The model under review builds one solid part; all positions refer to its coordinate system, in mm. Face numbers are marked on the shaded views. A direction names the side the tool comes from. Give positions to 0.01 mm unless a question says otherwise; leave off trailing zeros. Loops run counter-clockwise (first coordinate to the right, second up) from the corner with the lowest first, then second, coordinate; pieces in that order, holes last. Notation, with made-up numbers: (-3.75, -25) - (35.25, -25) arc R18 ccw to (35.25, 3) - close; hole circle Ø9 at (62.25, 27). An arc over 180 degrees is marked (long way). Answer as a JSON object with one key per item and string values.
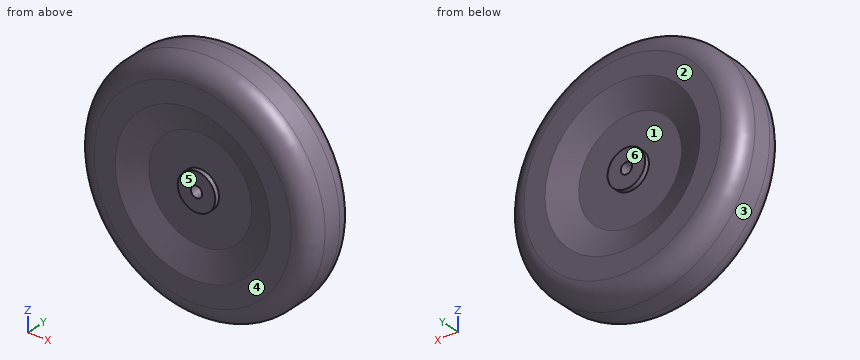
from build123d import *

# Parameters (mm, degrees)
F2_R = 20


with BuildPart() as f1:
    # F0 (on Right) → F1 (revolve)
    with BuildSketch(Plane.YZ):
        Polygon((-30, 82.617566), (-20, 54.791786), (-20, 20), (-25, 20), (-25, 6), (0, 6), (20, 6), (25, 6), (25, 20), (20, 20), (20, 54.791786), (30, 82.617566), (30, 125), (0, 125), (-30, 125), align=None)
    revolve(axis=Axis((0, 0.420819, 0), (0, 1, 0)))

    # F2
    f2_edges = [f1.edges().sort_by_distance(p)[0] for p in [
        (0, -30, -125),
        (0, 30, -125),
    ]]
    fillet(f2_edges, radius=F2_R)


solid = f1.part
Q1. The part is to be moulded in two halves that separate along X. For the marked faces 1, 2 and 3, say which applies: +X half, -X half, draft (parallel to the pull), parting line (faces both ways), or undercut.
Results:
{"face 1": "undercut", "face 2": "draft", "face 3": "parting line"}
Q2. Consider section A-A, the plane x = 0. State the section outline as (y, z) points, plus the area to 3 significant figures.
Results:
{"outline": "(-30, -105) arc R20 ccw to (-10, -125) - (10, -125) arc R20 ccw to (30, -105) - (30, -82.62) - (20, -54.79) - (20, -20) - (25, -20) - (25, -6) - (-25, -6) - (-25, -20) - (-20, -20) - (-20, -54.79) - (-30, -82.62) - close; (-30, 82.62) - (-20, 54.79) - (-20, 20) - (-25, 20) - (-25, 6) - (25, 6) - (25, 20) - (20, 20) - (20, 54.79) - (30, 82.62) - (30, 105) arc R20 ccw to (10, 125) - (-10, 125) arc R20 ccw to (-30, 105) - close", "area": "11,700 mm^2"}
Q3. For the marked faces 4, 5 and 6, list the 3-axis set-ups (+Z, -Z, +X, -X, +Y, -Y) from which the entire face can be reached by the end or side of a thin tool; tool diameter is ignored.
Results:
{"face 4": "+Z, -Z, +X, -X, -Y", "face 5": "-Y", "face 6": "+Y"}
Q4. Consider section B-B, the plane y = 4.5. State the section outline as (x, z) points.
Results:
{"outline": "circle Ø250 at (0, 0); hole circle Ø12 at (0, 0)"}
Q5. To check wall thickness, follow probe 1 along X at (y, z) = (-3.5, 0); probe 2 along X at (y, z) = (13.5, 0); probe 3 along Y at (x, z) = (-11, -7.5). State the ranges of each line that lie inside material, in increasing order. Write a range as [from, to].
Results:
{"probe 1": "x = [-125, -6], [6, 125]", "probe 2": "x = [-124.69, -6], [6, 124.69]", "probe 3": "y = [-25, 25]"}
Q6. Clearance check with flat-ended pins moving along their axes: pin 1 Ø20 at (x, z) = (-7, 3.5) entering from +Y; pin 2 Ø5 at (x, z) = (41, -59.5) entering from +Y; pin 3 Ø10 at (y, z) = (-22, -92.5) entering from -X; pin 4 Ø7 at (x, z) = (0, 0) entering from -Y. State where each tip first meets the part, or that it passes through.
Results:
{"pin 1": "stops at y = 25", "pin 2": "stops at y = 27.18", "pin 3": "stops at x = -85.22", "pin 4": "passes through"}
Q7. Consider section C-C, the plane y = -15. State the section outline as (x, z) points.
Results:
{"outline": "circle Ø248.73 at (0, 0); hole circle Ø12 at (0, 0)"}
